Check sheet for the modelled part. Datum: model origin and axes. Units: mm. Face numbers are marked on the shaded views. A direction names the side the tool comes from. Coordinates: 2 decimals unless noted, no trailing zeros. Loops run counter-clockwise (first coordinate to the right, second up) from the corner with the lowest first, then second, coordinate; pieces in that order, holes last. Notation, with made-up numbers: (-33, 62) - (-1, 62) arc R24 ccw to (-1, 75) - close; hole circle Ø1 at (56, 89). An arc over 180 degrees is marked (long way). Use a Markdown table: item, result. Add a question column.
1) Draft check along Z on the marked faces 4, 5 and 6. Enter one of: pulls with the +Z half, pulls with the -Z half, needs draft (parallel to the pull), parting line crosses it, or undercut.
2) Go/stop test with flat-tipped pins: P1, Ø2, axis at x = 1.5, y = 2, coming from the -Z side; P2, Ø1, axis at y = 1.5, z = 0, coming from the -X side; P3, Ø2, axis at x = 1, y = -2, coming from the +Z side. Record where each tip stops, or that it passes through.
3) Tool access check on the marked faces 1, 2 and 3. Record the directions out of +Z, -Z, +X, -X, +Y, -Y that give a thin tool (end or side, any length) a straight path to the whole face; none if there is none.
4) Sectioned sample at A-A, the plane x = 0. Enter the section's corners in (y, z).
5) Thickness scan on line 1 (X direction, y = 1.6, z = 2.75); line 2 (X direction, y = 2.4, z = 3); line 3 (Z direction, x = -1.25, y = 2.3). Record the ranges inside material, lowest first.
6) Sectioned sample at B-B, the plane x = -1.75. Enter the section's corners in (y, z).
from build123d import *

# Parameters (mm, degrees)
F0_R     = 1.58
F1_DEPTH = 3


with BuildPart() as f1:
    # F0 (on Front) → F1 (new body, symmetric)
    with BuildSketch(Plane.XZ):
        with BuildLine():
            ThreePointArc((0.1764835345, 2.6942259671), (0.1341691164, 2.7133752243), (0.1149463195, 2.7556562852))
            ThreePointArc((0.1149463195, 2.7556562852), (-0.0148204986, 3.3394100657), (-0.3129533658, 3.8577966946))
            ThreePointArc((-0.3129533658, 3.8577966946), (-0.3387771387, 3.8773936836), (-0.3708166587, 3.8823311303))
            ThreePointArc((-0.3708166587, 3.8823311303), (-0.5550278693, 3.8603036233), (-0.7379830973, 3.8295405662))
            ThreePointArc((-0.7379830973, 3.8295405662), (-0.7673337522, 3.8157765449), (-0.786590371, 3.789697974))
            ThreePointArc((-0.786590371, 3.789697974), (-0.9266003718, 3.2083159111), (-0.8866482769, 2.6116487228))
            ThreePointArc((-0.8866482769, 2.6116487228), (-0.8931804641, 2.5656646543), (-0.9283858818, 2.5353697274))
            ThreePointArc((-0.9283858818, 2.5353697274), (-1.1216205351, 2.4560063875), (-1.3081411324, 2.3619413155))
            ThreePointArc((-1.3081411324, 2.3619413155), (-1.7681239817, 2.0405238508), (-2.1517322648, 1.6309654382))
            ThreePointArc((-2.1517322648, 1.6309654382), (-2.2713845386, 1.4597302071), (-2.3774402326, 1.2797569848))
            ThreePointArc((-2.3774402326, 1.2797569848), (-2.5906310288, 0.7606779035), (-2.6919188572, 0.2087411462))
            ThreePointArc((-2.6919188572, 0.2087411462), (-2.7, 0), (-2.6919188572, -0.2087411462))
            ThreePointArc((-2.6919188572, -0.2087411462), (-2.5906310288, -0.7606779035), (-2.3774402326, -1.2797569848))
            ThreePointArc((-2.3774402326, -1.2797569848), (-2.2713845386, -1.4597302071), (-2.1517322648, -1.6309654382))
            ThreePointArc((-2.1517322648, -1.6309654382), (-1.7681239817, -2.0405238508), (-1.3081411324, -2.3619413155))
            ThreePointArc((-1.3081411324, -2.3619413155), (-1.1216205351, -2.4560063875), (-0.9283858818, -2.5353697274))
            ThreePointArc((-0.9283858818, -2.5353697274), (-0.3842500633, -2.6725178931), (0.1764835345, -2.6942259671))
            ThreePointArc((0.1764835345, -2.6942259671), (0.3842500633, -2.6725178931), (0.5897164591, -2.6348120422))
            ThreePointArc((0.5897164591, -2.6348120422), (1.1216205351, -2.4560063875), (1.6050759262, -2.1711129107))
            ThreePointArc((1.6050759262, -2.1711129107), (1.7681239817, -2.0405238508), (1.9205879909, -1.8977201503))
            ThreePointArc((1.9205879909, -1.8977201503), (2.2713845386, -1.4597302071), (2.5240680522, -0.9586868455))
            ThreePointArc((2.5240680522, -0.9586868455), (2.5906310288, -0.7606779035), (2.6416864059, -0.5581155194))
            ThreePointArc((2.6416864059, -0.5581155194), (2.7, 0), (2.6416864059, 0.5581155194))
            ThreePointArc((2.6416864059, 0.5581155194), (2.5906310288, 0.7606779035), (2.5240680522, 0.9586868455))
            ThreePointArc((2.5240680522, 0.9586868455), (2.2713845386, 1.4597302071), (1.9205879909, 1.8977201503))
            ThreePointArc((1.9205879909, 1.8977201503), (1.7681239817, 2.0405238508), (1.6050759262, 2.1711129107))
            ThreePointArc((1.6050759262, 2.1711129107), (1.1216205351, 2.4560063875), (0.5897164591, 2.6348120422))
            ThreePointArc((0.5897164591, 2.6348120422), (0.3842500633, 2.6725178931), (0.1764835345, 2.6942259671))
        make_face()
        Circle(F0_R, mode=Mode.SUBTRACT)
        with BuildLine():
            ThreePointArc((0.6660679051, 2.6764169638), (0.6357118151, 2.6412642707), (0.5897164591, 2.6348120422))
            ThreePointArc((0.5897164591, 2.6348120422), (1.1216205351, 2.4560063875), (1.6050759262, 2.1711129107))
            ThreePointArc((1.6050759262, 2.1711129107), (1.5798316425, 2.2100991926), (1.586519264, 2.256060913))
            ThreePointArc((1.586519264, 2.256060913), (1.7929535909, 2.8173030819), (1.822409234, 3.4145804618))
            ThreePointArc((1.822409234, 3.4145804618), (1.811279826, 3.4450278837), (1.7869958517, 3.4665034005))
            ThreePointArc((1.7869958517, 3.4665034005), (1.6201185507, 3.5475647819), (1.4495750544, 3.6205983154))
            ThreePointArc((1.4495750544, 3.6205983154), (1.4174423205, 3.6248874459), (1.3871434821, 3.6133596702))
            ThreePointArc((1.3871434821, 3.6133596702), (0.9550407005, 3.1999650771), (0.6660679051, 2.6764169638))
        make_face()
        with BuildLine():
            ThreePointArc((2.0073122334, 1.8914417294), (1.9627700848, 1.8782811435), (1.9205879909, 1.8977201503))
            ThreePointArc((1.9205879909, 1.8977201503), (2.2713845386, 1.4597302071), (2.5240680522, 0.9586868455))
            ThreePointArc((2.5240680522, 0.9586868455), (2.5239087847, 1.005132283), (2.554383552, 1.0401821415))
            ThreePointArc((2.554383552, 1.0401821415), (3.0314775838, 1.4007222756), (3.3791697785, 1.8872590586))
            ThreePointArc((3.3791697785, 1.8872590586), (3.3862682438, 1.9188900721), (3.3774498056, 1.9500853342))
            ThreePointArc((3.3774498056, 1.9500853342), (3.280888778, 2.1084991881), (3.1769033686, 2.2621416814))
            ThreePointArc((3.1769033686, 2.2621416814), (3.1521904717, 2.2831221951), (3.1204690807, 2.2898052019))
            ThreePointArc((3.1204690807, 2.2898052019), (2.5334630984, 2.175647941), (2.0073122334, 1.8914417294))
        make_face()
        with BuildLine():
            ThreePointArc((2.7112491106, 0.5059471103), (2.6666627208, 0.5189570245), (2.6416864059, 0.5581155194))
            ThreePointArc((2.6416864059, 0.5581155194), (2.7, 0), (2.6416864059, -0.5581155194))
            ThreePointArc((2.6416864059, -0.5581155194), (2.6666627208, -0.5189570245), (2.7112491106, -0.5059471103))
            ThreePointArc((2.7112491106, -0.5059471103), (3.3075288632, -0.4605779561), (3.8630677944, -0.2392537609))
            ThreePointArc((3.8630677944, -0.2392537609), (3.8861404204, -0.2164817791), (3.8955873101, -0.1854710471))
            ThreePointArc((3.8955873101, -0.1854710471), (3.9, 0), (3.8955873101, 0.1854710471))
            ThreePointArc((3.8955873101, 0.1854710471), (3.8861404204, 0.2164817791), (3.8630677944, 0.2392537609))
            ThreePointArc((3.8630677944, 0.2392537609), (3.3075288632, 0.4605779561), (2.7112491106, 0.5059471103))
        make_face()
        with BuildLine():
            ThreePointArc((-2.1517322648, 1.6309654382), (-1.7681239817, 2.0405238508), (-1.3081411324, 2.3619413155))
            ThreePointArc((-1.3081411324, 2.3619413155), (-1.3540911561, 2.3551737941), (-1.3931212693, 2.3803502573))
            ThreePointArc((-1.3931212693, 2.3803502573), (-1.8178891846, 2.8012779489), (-2.3489554831, 3.0761897348))
            ThreePointArc((-2.3489554831, 3.0761897348), (-2.3812747555, 3.0787143854), (-2.4108975001, 3.0655461575))
            ThreePointArc((-2.4108975001, 3.0655461575), (-2.5539568624, 2.94742334), (-2.69123683, 2.8226307454))
            ThreePointArc((-2.69123683, 2.8226307454), (-2.7084867804, 2.7951835518), (-2.7105873391, 2.7628339478))
            ThreePointArc((-2.7105873391, 2.7628339478), (-2.5140523732, 2.1980491121), (-2.1578598957, 1.7177004654))
            ThreePointArc((-2.1578598957, 1.7177004654), (-2.1384942569, 1.6754846382), (-2.1517322648, 1.6309654382))
        make_face()
        with BuildLine():
            ThreePointArc((2.554383552, -1.0401821415), (2.5239087847, -1.005132283), (2.5240680522, -0.9586868455))
            ThreePointArc((2.5240680522, -0.9586868455), (2.2713845386, -1.4597302071), (1.9205879909, -1.8977201503))
            ThreePointArc((1.9205879909, -1.8977201503), (1.9627700848, -1.8782811435), (2.0073122334, -1.8914417294))
            ThreePointArc((2.0073122334, -1.8914417294), (2.5334630984, -2.175647941), (3.1204690807, -2.2898052019))
            ThreePointArc((3.1204690807, -2.2898052019), (3.1521904717, -2.2831221951), (3.1769033686, -2.2621416814))
            ThreePointArc((3.1769033686, -2.2621416814), (3.280888778, -2.1084991881), (3.3774498056, -1.9500853342))
            ThreePointArc((3.3774498056, -1.9500853342), (3.3862682438, -1.9188900721), (3.3791697785, -1.8872590586))
            ThreePointArc((3.3791697785, -1.8872590586), (3.0314775838, -1.4007222756), (2.554383552, -1.0401821415))
        make_face()
        with BuildLine():
            ThreePointArc((-2.6919188572, 0.2087411462), (-2.5906310288, 0.7606779035), (-2.3774402326, 1.2797569848))
            ThreePointArc((-2.3774402326, 1.2797569848), (-2.4124370542, 1.2492213252), (-2.4588826984, 1.2492998415))
            ThreePointArc((-2.4588826984, 1.2492998415), (-3.043790899, 1.3737598761), (-3.6391808315, 1.3179142695))
            ThreePointArc((-3.6391808315, 1.3179142695), (-3.6677344627, 1.3025650229), (-3.6855354198, 1.2754719398))
            ThreePointArc((-3.6855354198, 1.2754719398), (-3.7420225971, 1.0987569717), (-3.7900418845, 0.9195556068))
            ThreePointArc((-3.7900418845, 0.9195556068), (-3.789714393, 0.8871395309), (-3.7739919791, 0.8587896644))
            ThreePointArc((-3.7739919791, 0.8587896644), (-3.3033105094, 0.4899172508), (-2.7439662444, 0.2783944468))
            ThreePointArc((-2.7439662444, 0.2783944468), (-2.704851233, 0.2533500879), (-2.6919188572, 0.2087411462))
        make_face()
        with BuildLine():
            ThreePointArc((1.586519264, -2.256060913), (1.5798316425, -2.2100991926), (1.6050759262, -2.1711129107))
            ThreePointArc((1.6050759262, -2.1711129107), (1.1216205351, -2.4560063875), (0.5897164591, -2.6348120422))
            ThreePointArc((0.5897164591, -2.6348120422), (0.6357118151, -2.6412642707), (0.6660679051, -2.6764169638))
            ThreePointArc((0.6660679051, -2.6764169638), (0.9550407005, -3.1999650771), (1.3871434821, -3.6133596702))
            ThreePointArc((1.3871434821, -3.6133596702), (1.4174423205, -3.6248874459), (1.4495750544, -3.6205983154))
            ThreePointArc((1.4495750544, -3.6205983154), (1.6201185507, -3.5475647819), (1.7869958517, -3.4665034005))
            ThreePointArc((1.7869958517, -3.4665034005), (1.811279826, -3.4450278837), (1.822409234, -3.4145804618))
            ThreePointArc((1.822409234, -3.4145804618), (1.7929535909, -2.8173030819), (1.586519264, -2.256060913))
        make_face()
        with BuildLine():
            ThreePointArc((-2.3774402326, -1.2797569848), (-2.5906310288, -0.7606779035), (-2.6919188572, -0.2087411462))
            ThreePointArc((-2.6919188572, -0.2087411462), (-2.704851233, -0.2533500879), (-2.7439662444, -0.2783944468))
            ThreePointArc((-2.7439662444, -0.2783944468), (-3.3033105094, -0.4899172508), (-3.7739919791, -0.8587896644))
            ThreePointArc((-3.7739919791, -0.8587896644), (-3.789714393, -0.8871395309), (-3.7900418845, -0.9195556068))
            ThreePointArc((-3.7900418845, -0.9195556068), (-3.7420225971, -1.0987569717), (-3.6855354198, -1.2754719398))
            ThreePointArc((-3.6855354198, -1.2754719398), (-3.6677344627, -1.3025650229), (-3.6391808315, -1.3179142695))
            ThreePointArc((-3.6391808315, -1.3179142695), (-3.043790899, -1.3737598761), (-2.4588826984, -1.2492998415))
            ThreePointArc((-2.4588826984, -1.2492998415), (-2.4124370542, -1.2492213252), (-2.3774402326, -1.2797569848))
        make_face()
        with BuildLine():
            ThreePointArc((0.1149463195, -2.7556562852), (0.1341691164, -2.7133752243), (0.1764835345, -2.6942259671))
            ThreePointArc((0.1764835345, -2.6942259671), (-0.3842500633, -2.6725178931), (-0.9283858818, -2.5353697274))
            ThreePointArc((-0.9283858818, -2.5353697274), (-0.8931804641, -2.5656646543), (-0.8866482769, -2.6116487228))
            ThreePointArc((-0.8866482769, -2.6116487228), (-0.9266003718, -3.2083159111), (-0.786590371, -3.789697974))
            ThreePointArc((-0.786590371, -3.789697974), (-0.7673337522, -3.8157765449), (-0.7379830973, -3.8295405662))
            ThreePointArc((-0.7379830973, -3.8295405662), (-0.5550278693, -3.8603036233), (-0.3708166587, -3.8823311303))
            ThreePointArc((-0.3708166587, -3.8823311303), (-0.3387771387, -3.8773936836), (-0.3129533658, -3.8577966946))
            ThreePointArc((-0.3129533658, -3.8577966946), (-0.0148204986, -3.3394100657), (0.1149463195, -2.7556562852))
        make_face()
        with BuildLine():
            ThreePointArc((-1.3081411324, -2.3619413155), (-1.7681239817, -2.0405238508), (-2.1517322648, -1.6309654382))
            ThreePointArc((-2.1517322648, -1.6309654382), (-2.1384942569, -1.6754846382), (-2.1578598957, -1.7177004654))
            ThreePointArc((-2.1578598957, -1.7177004654), (-2.5140523732, -2.1980491121), (-2.7105873391, -2.7628339478))
            ThreePointArc((-2.7105873391, -2.7628339478), (-2.7084867804, -2.7951835518), (-2.69123683, -2.8226307454))
            ThreePointArc((-2.69123683, -2.8226307454), (-2.5539568624, -2.94742334), (-2.4108975001, -3.0655461575))
            ThreePointArc((-2.4108975001, -3.0655461575), (-2.3812747555, -3.0787143854), (-2.3489554831, -3.0761897348))
            ThreePointArc((-2.3489554831, -3.0761897348), (-1.8178891846, -2.8012779489), (-1.3931212693, -2.3803502573))
            ThreePointArc((-1.3931212693, -2.3803502573), (-1.3540911561, -2.3551737941), (-1.3081411324, -2.3619413155))
        make_face()
    extrude(amount=F1_DEPTH, both=True)


solid = f1.part
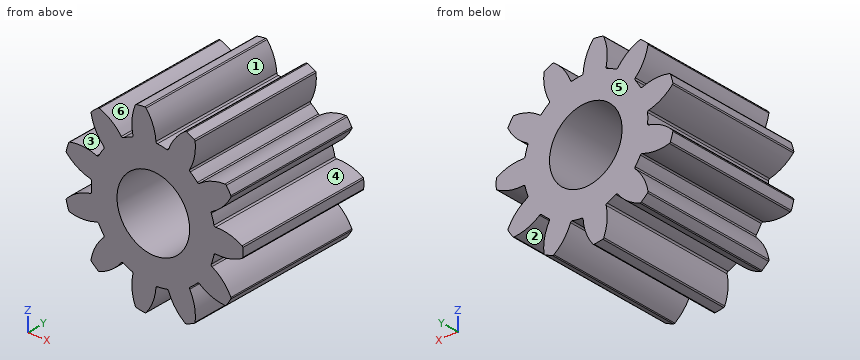
Solved:
| question | item | result |
|---|---|---|
| 1 | face 4 | undercut |
| 1 | face 5 | needs draft |
| 1 | face 6 | pulls with the +Z half |
| 2 | P1 | stops at z = -3.63 |
| 2 | P2 | stops at x = -3.32 |
| 2 | P3 | stops at z = 3.63 |
| 3 | face 1 | +Z, +Y, -Y |
| 3 | face 2 | -Z, +Y, -Y |
| 3 | face 3 | +Y, -Y |
| 4 | outline | (-3, -3.3) - (3, -3.3) - (3, -1.58) - (-3, -1.58) - close; (-3, 1.58) - (3, 1.58) - (3, 3.3) - (-3, 3.3) - close |
| 5 | line 1 | x = -2.71 to -1.75, -0.91 to 0.12, 0.69 to 1.78 |
| 5 | line 2 | x = -2.49 to -2.16, -0.93 to 0.08, 0.82 to 1.82 |
| 5 | line 3 | z = -2.39 to -0.97, 0.97 to 2.39 |
| 6 | outline | (-3, -2.75) - (3, -2.75) - (3, 2.75) - (-3, 2.75) - close |
